Design review of the part built by this model. Coordinates are the model's own, in mm. Coordinates: 2 decimals unless noted, no trailing zeros. Write each loop counter-clockwise with the first axis right and the second up, starting at its lowest first coordinate (ties: lowest second). Pieces come first, ordered by that corner, then holes.
Autodesk Inventor part; units mm, degrees
ref_plane "YZ Plane" through (0, 0, 0) normal (1, 0, 0) x (0, 1, 0)
ref_plane "XZ Plane" through (0, 0, 0) normal (0, 1, 0) x (-1, 0, 0)
ref_plane "XY Plane" through (0, 0, 0) normal (0, 0, 1) x (1, 0, 0)
sketch "Sketch1" plane through (0, 0, 0) normal (0, 0, 1) x (1, 0, 0)
  line L0 (-15.2, 0) -> (15.2, 0) construction
  arc A0 (-12.7505, 2.5) -> (-12.7505, -2.5) centre (-15.2, 0) ccw
  arc A1 (12.7505, -2.5) -> (12.7505, 2.5) centre (15.2, 0) ccw
  line L1 (-12.7505, 2.5) -> (12.7505, 2.5)
  line L2 (12.7505, -2.5) -> (-12.7505, -2.5)
  point P0 (0, 0)
  point P1 (0, 0)
  dimension "d0" = 3.5
  dimension "d1" = 30.4
  dimension "d26" = 3.5
  dimension "d27" = 5
extrude "Extrusion1" add sketch "Sketch1" along normal blind 1.5
hole "Hole1" at (-15.2, 0, 1.5) direction (0, 0, -1) diameter 5 end through all
hole "Hole2" at (15.2, 0, 1.5) direction (0, 0, -1) diameter 5 end through all
fillet "Fillet1" radius 3 4 edges at (-12.7505, -2.5, 0.75) (12.7505, -2.5, 0.75) (12.7505, 2.5, 0.75) (-12.7505, 2.5, 0.75)
properties part number "tendon"
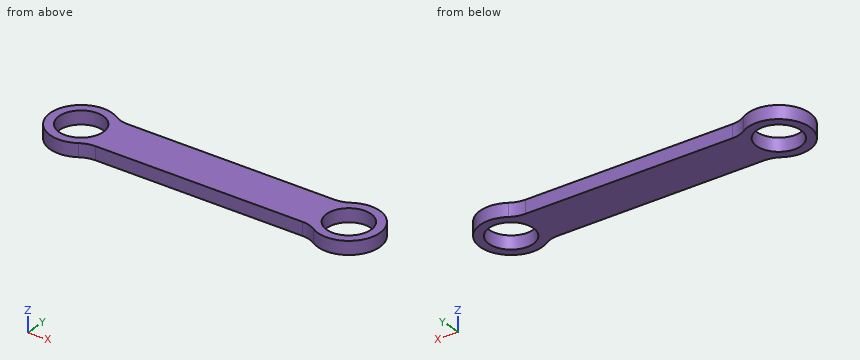
(1) Consider section B-B (x = 15.2). Give the boundary of the cut face in (y, z).
(2) Wall thickness on line 1 (X direction, y = 0, z = 1.05); line 2 (Y direction, x = 15.2, z = 0.95); line 3 (X direction, y = -0.5, z = 1.15): over which ranges is each line inside the solid? List them lowest first.
(3) Consider section A-A (z = 1.1). Give the boundary of the cut face in (x, y), plus the area to 3 significant figures.
(4) Consider section C-C (y = 0.5). Give the boundary of the cut face in (x, z).
(5) Consider section D-D (x = 10). Give the boundary of the cut face in (y, z).
Results:
1. outline: (-3.5, 0) - (-2.5, 0) - (-2.5, 1.5) - (-3.5, 1.5) - close; (2.5, 0) - (3.5, 0) - (3.5, 1.5) - (2.5, 1.5) - close
2. line 1: x = -18.7 to -17.7, -12.7 to 12.7, 17.7 to 18.7
2. line 2: y = -3.5 to -2.5, 2.5 to 3.5
2. line 3: x = -18.66 to -17.65, -12.75 to 12.75, 17.65 to 18.66
3. outline: (-13.33, -2.96) arc R3 cw to (-11.74, -2.5) - (11.74, -2.5) arc R3 cw to (13.33, -2.96) arc R3.5 ccw (long way) to (13.33, 2.96) arc R3 cw to (11.74, 2.5) - (-11.74, 2.5) arc R3 cw to (-13.33, 2.96) arc R3.5 ccw (long way) to start; hole circle Ø5 at (-15.2, 0); hole circle Ø5 at (15.2, 0)
3. area: 158 mm2
4. outline: (-18.66, 0) - (-17.65, 0) - (-17.65, 1.5) - (-18.66, 1.5) - close; (-12.75, 0) - (12.75, 0) - (12.75, 1.5) - (-12.75, 1.5) - close; (17.65, 0) - (18.66, 0) - (18.66, 1.5) - (17.65, 1.5) - close
5. outline: (-2.5, 0) - (2.5, 0) - (2.5, 1.5) - (-2.5, 1.5) - close
